Autodesk Fusion 360 part; units mm, degrees
sketch "Sketch1" plane through (0, 0, 0) normal (0, 1, 0) x (1, 0, 0)
  line L0 (50, 30) -> (-50, 30)
  line L1 (-50, 30) -> (-50, -30)
  line L2 (-50, -30) -> (50, -30)
  line L3 (50, -30) -> (50, 30)
  line L4 (50, 30) -> (-50, -30) construction
  line L5 (-50, 30) -> (50, -30) construction
  dimension "d1" = 100
  dimension "d2" = 60
extrude "Extrude1" add sketch "Sketch1" along normal blind 30
sketch "Sketch2" plane through (0, 0, 0) normal (0, 1, 0) x (1, 0, 0)
  circle A0 centre (0, 0) radius 25
  dimension "d5" = 50
extrude "Extrude2" add sketch "Sketch2" against normal blind 20
sketch "Sketch3" plane through (0, 0, 0) normal (0, -1, 0) x (1, 0, 0)
  circle A0 centre (0, 0) radius 25
  line L0 (50, -30) -> (50, 30)
  line L1 (50, 30) -> (-50, 30)
  line L2 (-50, 30) -> (-50, -30)
  line L3 (-50, -30) -> (50, -30)
sketch "Sketch4" plane through (0, 0, 30) normal (0, 0, 1) x (-1, 0, 0)
  line L0 (50, 0) -> (-50, 0)
  line L1 (-50, 0) -> (-50, -30)
  line L2 (-50, -30) -> (50, -30)
  line L3 (50, -30) -> (50, 0)
  circle A0 centre (-35, -15) radius 10
  line L4 (42.5777, -25.1555) -> (27.5777, -25.1555)
  line L5 (27.5777, -25.1555) -> (27.5777, -10.1555)
  line L6 (27.5777, -10.1555) -> (42.5777, -10.1555)
  line L7 (42.5777, -10.1555) -> (42.5777, -25.1555)
  dimension "d8" = 20
  dimension "d9" = 15
  dimension "d10" = 15
extrude "Extrude3" add sketch "Sketch4" along normal blind 5 contours A0
sketch "Sketch5" plane through (0, 0, 30) normal (0, 0, 1) x (-1, 0, 0)
  circle A0 centre (-35, -15) radius 10
  line L0 (50, 0) -> (-50, 0)
  line L1 (-50, 0) -> (-50, -30)
  line L2 (-50, -30) -> (50, -30)
  line L3 (50, -30) -> (50, 0)
  line L4 (45.1493, -24.9291) -> (30.1493, -24.9291)
  line L5 (30.1493, -24.9291) -> (30.1493, -9.9291)
  line L6 (30.1493, -9.9291) -> (45.1493, -9.9291)
  line L7 (45.1493, -9.9291) -> (45.1493, -24.9291)
  dimension "d13" = 15
  dimension "d14" = 15
extrude "Extrude4" add sketch "Sketch5" along normal blind 5 contours L4 L5 L6 L7
sketch "Sketch6" plane through (0, 0, 30) normal (0, 0, 1) x (-1, 0, 0)
  line L0 (45.1493, -9.9291) -> (45.1493, -24.9291)
  line L1 (45.1493, -24.9291) -> (30.1493, -24.9291)
  line L2 (30.1493, -24.9291) -> (30.1493, -9.9291)
  line L3 (30.1493, -9.9291) -> (45.1493, -9.9291)
  circle A0 centre (-35, -15) radius 10
  line L4 (50, 0) -> (-50, 0)
  line L5 (-50, 0) -> (-50, -30)
  line L6 (-50, -30) -> (50, -30)
  line L7 (50, -30) -> (50, 0)
box "BoxPrimitive1" add length 30 width 30 height 10 placed x (0, -1, 0) y (1, 0, 0) z (0, 0, 1) at (-15, 30, 30)
chamfer "Chamfer1" distance 10 angle 45 1 edges at (0, 0, 40)
CAD build for the part. Positions are in the model's coordinates, mm. A direction names the side the tool comes from. Coordinates: 2 decimals unless noted, no trailing zeros. Order: outer loops, then holes, each group sorted by start corner. A loop starts at its lowest first (then second) coordinate and runs counter-clockwise, first axis right, second up.
(1) Drill centre lines: L1, parallel to Y at x = -31.5, z = -2; L2, parallel to Z at x = -35, y = 22; L3, parallel to Z at x = -39.5, y = 6. Where is each one in solid material? Low to high.
Solution:
L1: y = 0 to 30
L2: z = -30 to 35
L3: z = -30 to 30
(2) Saw through at B-B, the plane y = 15. Write the cut outline in (x, z).
Solution:
outline: (-50, -30) - (50, -30) - (50, 30) - (45, 30) - (45, 35) - (25, 35) - (25, 30) - (15, 30) - (15, 40) - (-15, 40) - (-15, 30) - (-30.15, 30) - (-30.15, 35) - (-45.15, 35) - (-45.15, 30) - (-50, 30) - close
(3) Pin check, flat tips, straight feed: pin 1 Ø8 at (y, z) = (10.5, 37) entering from -X; pin 2 Ø1 at (x, z) = (-28, 7.5) entering from -Y; pin 3 Ø15 at (x, y) = (-39.5, 21) entering from +Z. Stop position of each tip, or through.
Solution:
pin 1: stops at x = -45.15
pin 2: stops at y = 0
pin 3: stops at z = 35
(4) Mould opens along X. For faces 1 (the face through (23.846, -9.86, -7.509)), 2 (the face through (0, 20, 40)), 3 (the face through (42.37, 21.76, 32.47)) say: released by +X, released by -X, zero draft, split by the parting line, or undercut.
Solution:
face 1: split by the parting line
face 2: zero draft
face 3: undercut
(5) Saw through at C-C, the plane z = 0. Write the cut outline in (x, y).
Solution:
outline: (-50, 0) - (-25, 0) - (-25, -20) - (25, -20) - (25, 0) - (50, 0) - (50, 30) - (-50, 30) - close
(6) Saw through at A-A, the plane x = 35. Write the cut outline in (y, z).
Solution:
outline: (0, -30) - (30, -30) - (30, 30) - (25, 30) - (25, 35) - (5, 35) - (5, 30) - (0, 30) - close
(7) Which spindle directions (+Z, -Z, +X, -X, +Y, -Y) get a long thin tool onto all of the face, cutting with end or side? Do faces 4 (the face through (35, 15, 35)), 5 (the face through (-38, 24.929, 32)), 6 (the face through (15, 18, 35)). Say none if no direction does.
Solution:
face 4: +Z, +X, +Y, -Y
face 5: +Z, -X, +Y
face 6: +Z, +Y, -Y
(8) Saw through at D-D, the plane x = 0. Write the cut outline in (y, z).
Solution:
outline: (-20, -25) - (0, -25) - (0, -30) - (30, -30) - (30, 40) - (10, 40) - (0, 30) - (0, 25) - (-20, 25) - close
